Source: CAD feature listing. Evaluate the final solid. Frame: model axes, mm. A direction names the side the tool comes from. Give positions to 0.01 mm unless a question says otherwise; leave off trailing zeros. Loops run counter-clockwise (first coordinate to the right, second up) from the corner with the lowest first, then second, coordinate; pieces in that order, holes last. Notation, with made-up numbers: (78, -29.5) -> (84, -29.5) arc R10 ccw to (84, -16.5) -> close; hole circle Ø4 at (-32, -32). An arc over 180 degrees is marked (long way). Return JSON: item names as keys, results as strings. Group by question number.
(1) Cut plane D-D on y = 0. Return loops of the section in (x, z), then the cut area to 3 significant figures.
(2) Draft query along Y for faces 5 (the face through (-0.13, 30.46, 0.59)), 6 (the face through (0.035, 22.258, -11.748)), 7 (the face through (9.5, 26, -5)). Return one class per face: released by +Y, released by -Y, zero draft, split by the parting line, or undercut.
(3) Ray query, line 1 (Y direction, x = -5.25, z = 5); line 2 (X direction, y = 0, z = 6.5); line 3 (Y direction, x = 4.75, z = 1). Return the intervals inside material, ascending. Write a range as from..to.
(4) Cut plane A-A on x = 0. Return loops of the section in (y, z), then the cut area to 3 significant figures.
(5) Access query for faces 1 (the face through (-9.5, 26, -5)), 2 (the face through (2.5, 18, 8)), 3 (the face through (2.5, 18, -8)), 4 (the face through (-2.5, 18, 0)). Directions: +Z, -Z, +X, -X, +Y, -Y. A direction counts if a zero-diameter tool reaches every point of the face in a straight line with its end or side. Return the directions, or none.
(6) Cut plane C-C on x = -3.75. Return loops of the section in (y, z), then the cut area to 3 significant figures.
(7) Cut plane B-B on z = 0. Return loops of the section in (x, y), then the cut area to 3 significant figures.
(8) Pin query (flat end, axial travel): pin 1 (4 mm diameter, centred on x = 6, y = 23.5, fed in from -Z); pin 2 (2 mm diameter, centred on y = 3, z = -2.5, fed in from +X); pin 3 (7.5 mm diameter, centred on y = 28, z = -3, fed in from -X). Return the tip coordinate at first contact, or that it passes through.
```python
from build123d import *

# Parameters (mm, degrees)
SKETCH1_R               = 14
BOSS_EXTRUDE1_DEPTH     = 17.5
CUT_EXTRUDE1_DEPTH      = 27.424420523
CUT_EXTRUDE1_DEPTH_BACK = 27.424420523
SKETCH2_R               = 9
SKETCH3_R               = 7.5
BOSS_EXTRUDE2_DEPTH     = 9.5
CUT_EXTRUDE2_DEPTH      = 45.505617623
CUT_EXTRUDE2_DEPTH_BACK = 45.505617623
SKETCH4_R               = 4.5
BOSS_EXTRUDE3_DEPTH     = 2.5
RIB3_START              = -2.5
RIB3_DEPTH              = 5


with BuildPart() as part:
    # Sketch1 → Boss-Extrude1 (new, symmetric)
    with BuildSketch(Plane.XY):
        Circle(SKETCH1_R)
    extrude(amount=BOSS_EXTRUDE1_DEPTH, both=True)

    # Sketch2 → Cut-Extrude1 (cut, two sides: drawn at the far end of the back side and taken through both)
    with BuildSketch(Plane.XY.offset(-CUT_EXTRUDE1_DEPTH_BACK)):
        Circle(SKETCH2_R)
    extrude(amount=CUT_EXTRUDE1_DEPTH + CUT_EXTRUDE1_DEPTH_BACK, mode=Mode.SUBTRACT)



with BuildPart() as body_2:
    # Sketch3 → Boss-Extrude2 (new, symmetric)
    with BuildSketch(Plane(origin=(0, 0, 0), x_dir=(0, 0, -1), z_dir=(1, 0, 0))):
        with Locations((0, 26)):
            Circle(SKETCH3_R)
    extrude(amount=BOSS_EXTRUDE2_DEPTH, both=True)

    # Sketch4 → Cut-Extrude2 (cut, two sides: drawn at the far end of the back side and taken through both)
    with BuildSketch(Plane(origin=(9.5, 0, 0), x_dir=(0, 0, -1), z_dir=(1, 0, 0)).offset(-CUT_EXTRUDE2_DEPTH_BACK)):
        with Locations((0, 26)):
            Circle(SKETCH4_R)
    extrude(amount=CUT_EXTRUDE2_DEPTH + CUT_EXTRUDE2_DEPTH_BACK, mode=Mode.SUBTRACT)


with BuildPart() as part_1:
    add(part.part)

    add(body_2.part)  # Boss-Extrude3 merges body 2
    # Sketch5 → Boss-Extrude3 (add, symmetric)
    with BuildSketch(Plane(origin=(0, 0, 0), x_dir=(0, 0, -1), z_dir=(1, 0, 0))):
        with BuildLine():
            Line((-17.5, 14), (-6.153967777, 30.287036342))
            ThreePointArc((-6.153967777, 30.287036342), (-7.414340436, 27.130290186), (-7.151829247, 23.741385731))
            ThreePointArc((-7.151829247, 23.741385731), (-4.43341815, 19.950636107), (0, 18.5))
            ThreePointArc((0, 18.5), (4.056082014, 19.691418646), (6.823499563, 22.887147015))
            ThreePointArc((6.823499563, 22.887147015), (7.328923752, 24.407242442), (7.5, 26))
            ThreePointArc((7.5, 26), (7.155583775, 28.246691086), (6.153967777, 30.287036342))
            Line((6.153967777, 30.287036342), (17.5, 14))
            Line((17.5, 14), (17.5, 12.5))
            Line((17.5, 12.5), (-17.5, 12.5))
            Line((-17.5, 12.5), (-17.5, 14))
        make_face()
    extrude(amount=BOSS_EXTRUDE3_DEPTH, both=True)

    # Rib3: read off the stored shape, not the designer's step
    # Rib3 outline → Rib3 (add)
    with BuildSketch(Plane.XY.offset(RIB3_START)):
        with BuildLine():
            Line((9.5, 18.928932188), (2.5, 18.928932188))
            Line((2.5, 18.928932188), (2.5, 13.774977314))
            ThreePointArc((2.5, 13.774977314), (9.472147799, 10.309142354), (13.514557534, 3.654686672))
            Line((13.514557534, 3.654686672), (9.5, 18.5))
            Line((9.5, 18.5), (9.5, 18.928932188))
        make_face()
    extrude(amount=RIB3_DEPTH)


solid = part_1.part
```
Answers:
{
 "1": {"outline": "(-14, -17.5) -> (-9, -17.5) -> (-9, 17.5) -> (-14, 17.5) -> close; (9, -17.5) -> (14, -17.5) -> (14, 17.5) -> (9, 17.5) -> close", "area": "350 mm²"},
 "2": {"face 5": "undercut", "face 6": "released by +Y", "face 7": "zero draft"},
 "3": {"line 1": "-12.98..-7.31, 7.31..12.98, 20.41..31.59", "line 2": "-14..-9, 9..14", "line 3": "-13.17..-7.64, 7.64..21.61, 30.39..33.43"},
 "4": {"outline": "(-14, -17.5) -> (-9, -17.5) -> (-9, 17.5) -> (-14, 17.5) -> close; (9, -17.5) -> (14, -17.5) -> (30.29, -6.15) arc R7.5 ccw to (30.29, 6.15) -> (14, 17.5) -> (9, 17.5) -> close; hole circle Ø9 at (26, 0)", "area": "699 mm²"},
 "5": {"face 1": "+Z, -Z, -X, +Y", "face 2": "+Z, +X", "face 3": "-Z, +X", "face 4": "-X"},
 "6": {"outline": "(-13.49, -17.5) -> (-8.18, -17.5) -> (-8.18, 17.5) -> (-13.49, 17.5) -> close; (8.18, -17.5) -> (13.49, -17.5) -> (13.49, 17.5) -> (8.18, 17.5) -> close; circle Ø15 at (26, 0); hole circle Ø9 at (26, 0)", "area": "485 mm²"},
 "7": {"outline": "(-9.5, 18.5) -> (-2.5, 18.5) -> (-2.5, 13.77) arc R14 ccw (long way) to (13.51, 3.65) -> (9.5, 18.5) -> (9.5, 21.5) -> (-9.5, 21.5) -> close; (-9.5, 30.5) -> (9.5, 30.5) -> (9.5, 33.5) -> (-9.5, 33.5) -> close; hole circle Ø18 at (0, 0)", "area": "554 mm²"},
 "8": {"pin 1": "z = -7.48", "pin 2": "x = 13.86", "pin 3": "x = -9.5"}
}
